```python
from build123d import *

# Parameters (mm, degrees)
CUT_EXTRUDE_1_DEPTH      = 96.262794416
CUT_EXTRUDE_1_DEPTH_BACK = 96.262794416
SKETCH_2_W               = 55
SKETCH_2_H               = 110
CUT_EXTRUDE_2_DEPTH      = 96.262794416
CUT_EXTRUDE_2_DEPTH_BACK = 96.262794416
SKETCH_3_W               = 23.273135213
SKETCH_3_H               = 110
CUT_EXTRUDE_3_DEPTH      = 87.788536109
SKETCH_5_W               = 1
SKETCH_5_H               = 20
CUT_EXTRUDE_4_DEPTH      = 87.788536109
SKETCH_6_W               = 11.3
SKETCH_6_H               = 3.5
CUT_EXTRUDE_START        = -10
CUT_EXTRUDE_5_DEPTH      = 10
SKETCH_8_W               = 49.8
SKETCH_8_H               = 41.258728368
CUT_EXTRUDE_7_DEPTH      = 99.910110707
CUT_EXTRUDE_8_DEPTH      = 70
CUT_EXTRUDE_8_DEPTH_BACK = 70
CUT_EXTRUDE_9_DEPTH      = 70


with BuildPart() as part:
    # Sketch 1 → Revolve 8 (revolve)
    with BuildSketch(Plane.XY):
        with BuildLine():
            Line((0, 55), (0, 51.5))
            ThreePointArc((0, 51.5), (-51.5, 0), (0, -51.5))
            Line((0, -51.5), (0, -55))
            ThreePointArc((0, -55), (-55, 0), (0, 55))
        make_face()
    revolve(axis=Axis((0, 0, 0), (0, 1, 0)))

    # Sketch 2 → Cut-Extrude 1 (cut, two sides: drawn at the far end of the back side and taken through both)
    with BuildSketch(Plane.XY.offset(-CUT_EXTRUDE_1_DEPTH_BACK)):
        with Locations((27.5, 0)):
            Rectangle(SKETCH_2_W, SKETCH_2_H)
    extrude(amount=CUT_EXTRUDE_1_DEPTH + CUT_EXTRUDE_1_DEPTH_BACK, mode=Mode.SUBTRACT)

    # Sketch 3 → Cut-Extrude 2 (cut, two sides: drawn at the far end of the back side and taken through both)
    with BuildSketch(Plane.XY.offset(-CUT_EXTRUDE_2_DEPTH_BACK)):
        with Locations((-50.136567607, 0)):
            Rectangle(SKETCH_3_W, SKETCH_3_H)
    extrude(amount=CUT_EXTRUDE_2_DEPTH + CUT_EXTRUDE_2_DEPTH_BACK, mode=Mode.SUBTRACT)

    # Sketch 4 → Cut-Extrude 3 (cut, through all)
    with BuildSketch(Plane.ZY.offset(38.5)):
        with BuildLine():
            Line((0, 0), (0, 64.529887393))
            ThreePointArc((0, 64.529887393), (-55.884521786, -32.264943697), (55.884521786, -32.264943697))
            Line((55.884521786, -32.264943697), (0, 0))
        make_face()
    extrude(amount=-CUT_EXTRUDE_3_DEPTH, mode=Mode.SUBTRACT)

    # Sketch 5 → Cut-Extrude 4 (cut, through all)
    with BuildSketch(Plane(origin=(0, 0, 0), x_dir=(-1, 0, 0), z_dir=(0, 0, -1))):
        with Locations((31, 45)):
            Rectangle(SKETCH_5_W, SKETCH_5_H)
        with Locations((10.5, 45)):
            Rectangle(SKETCH_5_W, SKETCH_5_H)
    extrude(amount=-CUT_EXTRUDE_4_DEPTH, mode=Mode.SUBTRACT)

    # Sketch 6 → Revolve 9 (revolve)
    with BuildSketch(Plane.XY, mode=Mode.PRIVATE) as revolve_9_sk:
        with Locations((5.65, 53.25)):
            Rectangle(SKETCH_6_W, SKETCH_6_H)
    revolve(revolve_9_sk.sketch.rotate(Axis((0, 0, 0), (1, 0, 0)), 90), axis=Axis((0, 0, 0), (1, 0, 0)))

    # Sketch 7 → Cut-Extrude 5 (cut)
    with BuildSketch(Plane.ZY.offset(CUT_EXTRUDE_START)):
        with BuildLine():
            Line((0, 55), (0, 0))
            Line((0, 0), (47.631397208, -27.5))
            ThreePointArc((47.631397208, -27.5), (-47.631397208, -27.5), (0, 55))
        make_face()
    extrude(amount=CUT_EXTRUDE_5_DEPTH, mode=Mode.SUBTRACT)

    # Mirror 1: part across plane


with BuildPart() as part_1:
    add(part.part)
    add(part.part.mirror(Plane(origin=(11.3, 55, 0), x_dir=(0, 0, 1), z_dir=(-1, 0, 0))))

    # Sketch 8 → Cut-Extrude 7 (cut, through all)
    with BuildSketch(Plane.XY):
        Polygon((-38.5, 54.805759265), (-38.5, 9.819464089), (11.3, 9.819464089), (11.3, 56.704937245), align=None)
        with Locations((-13.6, -10.809900095)):
            Rectangle(SKETCH_8_W, SKETCH_8_H)
    extrude(amount=CUT_EXTRUDE_7_DEPTH, mode=Mode.SUBTRACT)

    # Sketch 9 → Cut-Extrude 8 (cut, two sides: drawn at the far end of the back side and taken through both)
    with BuildSketch(Plane.XY.offset(-CUT_EXTRUDE_8_DEPTH_BACK)):
        Polygon((11.3, 55), (11.3, 58.911756152), (4.567331784, 58.911756152), (4.567331784, -60.848172915), (11.3, -60.848172915), align=None)
    extrude(amount=CUT_EXTRUDE_8_DEPTH + CUT_EXTRUDE_8_DEPTH_BACK, mode=Mode.SUBTRACT)

    # Sketch 10 → Cut-Extrude 9 (cut)
    with BuildSketch(Plane(origin=(12.6, 0, 0), x_dir=(0, 0, -1), z_dir=(1, 0, 0))):
        with BuildLine():
            Line((0, 55), (0, 0))
            Line((0, 0), (-47.631397208, -27.5))
            ThreePointArc((-47.631397208, -27.5), (47.631397208, -27.5), (0, 55))
        make_face()
    extrude(amount=-CUT_EXTRUDE_9_DEPTH, mode=Mode.SUBTRACT)


solid = part_1.part
```
Model file for the job. Use its own axes, mm. A direction names the side the tool comes from. Coordinates: 2 decimals unless noted, no trailing zeros. Order: outer loops, then holes, each group sorted by start corner. A loop starts at its lowest first (then second) coordinate and runs counter-clockwise, first axis right, second up. Notation, with made-up numbers: (-1, 72.5) - (7, 72.5) arc R29 ccw to (7, 108.5) - close; hole circle Ø11 at (87.25, 28.5). An arc over 180 degrees is marked (long way). Return JSON: item names as keys, results as strings. Group by question number.
1) Saw through at B-B, the plane z = 24.5. Write the cut outline in (x, y).
2) Tool access for faces 1 (the flat face through (54.1, 40, 14)), 2 (the flat face through (22, 53, 0)), 3 (the cylindrical face through (16.87, 26.4, 44.22)): list every direction of +Z, -Z, +X, -X, +Y, -Y with a clear straight run to the whole face (end or side of a thin tool).
3) Flat gauge pins, fed straight in: P1, Ø0.5, axis at x = 53.5, z = 23, coming from the +Y side; P2, Ø5, axis at x = 54.5, z = 40, coming from the -Y side; P3, Ø10, axis at x = 54.5, z = 44.5, coming from the +Y side (3 decimals); P4, Ø12, axis at y = 38.5, z = 9, coming from the +X side. Where does each tip first touch, or does it go through?
4) Mould opens along X. For faces 4 (the flat face through (43, 49, 0)), 5 (the flat face through (33.6, 47, 20)), 6 (the flat face through (11.3, 26, 46)) say: released by +X, released by -X, zero draft, split by the parting line, or undercut.
5) Saw through at C-C, the plane y = 9. Write the cut outline in (x, z), plus the area to 3 significant figures.
6) Probe line 1 (X direction, y = 44, z = 4); line 2 (Y direction, x = 56.5, z = 14); line 3 (Y direction, x = 33.5, z = 45.5). List the from-to ranges inside material, lowest first. Write a range as from..to.
7) Saw through at D-D, the plane z = 50. Write the cut outline in (x, y).
8) Saw through at A-A, the plane z = 18.5. Write the cut outline in (x, y).
Values found:
{
 "1": {"outline": "(11.3, 45.3) - (22.6, 45.3) arc R45.3 cw to (32.6, 44.18) - (32.6, 48.22) arc R49.24 ccw to (22.6, 49.24) - (11.3, 49.24) - close; (33.6, 43.94) arc R45.3 cw to (61.1, 23.87) - (61.1, 30.7) arc R49.24 ccw to (54.1, 37.85) - (54.1, 35) - (53.1, 35) - (53.1, 38.66) arc R49.24 ccw to (33.6, 48) - close"},
 "2": {"face 1": "+Z, -Z, +Y", "face 2": "-Z, +X, -X, +Y, -Y", "face 3": "-Z, -X"},
 "3": {"P1": "stops at y = 35", "P2": "stops at y = -23.24", "P3": "stops at y = 23.445", "P4": "stops at x = 61.1"},
 "4": {"face 4": "zero draft", "face 5": "undercut", "face 6": "released by -X"},
 "5": {"outline": "(11.3, 50.71) - (22.6, 50.71) arc R50.71 cw to (61.1, 33) - (61.1, 38.23) arc R54.26 ccw to (22.6, 54.26) - (11.3, 54.26) - close", "area": "194 mm²"},
 "6": {"line 1": "x = 49.06..53.1, 54.1..55.36", "line 2": "y = 36.15..40.99", "line 3": "y = -26.27..-21.52, 21.52..28.91"},
 "7": {"outline": "(11.3, -22.91) - (22.6, -22.91) arc R22.91 ccw to (22.6, 22.91) - (11.3, 22.91) - (11.3, 12.34) - (22.6, 12.34) arc R12.34 cw to (22.6, -12.34) - (11.3, -12.34) - close"},
 "8": {"outline": "(11.3, 48.06) - (22.6, 48.06) arc R48.06 cw to (32.6, 47.01) - (32.6, 50.82) arc R51.8 ccw to (22.6, 51.8) - (11.3, 51.8) - close; (33.6, 46.79) arc R48.06 cw to (53.1, 37.14) - (53.1, 41.86) arc R51.8 ccw to (33.6, 50.61) - close; (54.1, 36.3) arc R48.06 cw to (61.1, 28.77) - (61.1, 34.65) arc R51.8 ccw to (54.1, 41.12) - close"}
}
